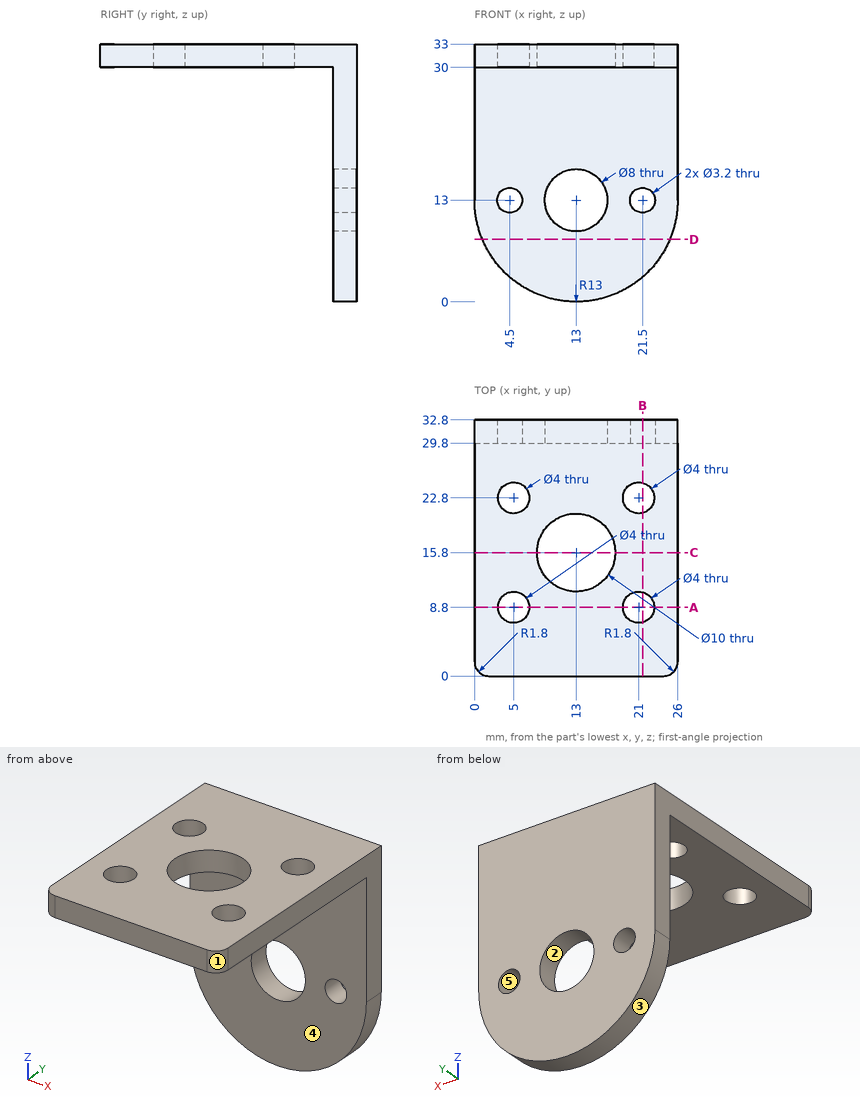
Check sheet for the drawn part. Datum: minimum x, y, z corner. Units: mm. A direction names the side the tool comes from. Coordinates: 2 decimals unless noted, no trailing zeros. Order: outer loops, then holes, each group sorted by start corner. A loop starts at its lowest first (then second) coordinate and runs counter-clockwise, first axis right, second up. Notation, with made-up numbers: M 75.5,-10.5 L 98.5,-10.5 A34 cw 98.5,23.5 Z; hole C 52,6.5 d8. An arc over 180 degrees is marked long. One line per question, with ' | ' between items. Start each with the question number.
Item 1: Access from +Z, -Z, +X, -X, +Y, -Y to the whole of each face (thin tool, end or side, straight path). Record for the marked faces 4 and 5.
Item 2: Gauge pin test, flat ends, axial feed: P1, Ø3.5, axis at x = 21.5, z = 13, coming from the -Y side; P2, Ø11.5, axis at x = 13, y = 15.8, coming from the -Z side; P3, Ø8, axis at x = 20, y = 28.5, coming from the -Z side. Record the tip position at first contact, or that the pin passes through.
Item 3: Sectioned sample at A-A on y = 8.8. Record the cut outline in (x, z).
Item 4: Mould release check, pull along Z, two halves, no side actions. Record for the marked faces 1, 2 and 3: pulls with the +Z half, pulls with the -Z half, needs draft (parallel to the pull), parting line crosses it, or undercut.
Item 5: Sectioned sample at C-C on y = 15.8. Record the cut outline in (x, z), and give its area (3 significant figures).
Item 6: Sectioned sample at B-B on x = 21.5. Record the cut outline in (y, z).
Item 7: Material ranges on line 1 (Y direction, x = 5, z = 32.3); line 2 (Y direction, x = 13, z = 30.75); line 3 (X direction, y = 8, z = 32), recorded low to high.
Item 8: Sectioned sample at D-D on z = 8. Record the cut outline in (x, y).
Answer below:
1) face 4: -Z, +X, -X, -Y | face 5: +Y, -Y
2) P1: stops at y = 29.8 | P2: stops at z = 30 | P3: stops at z = 0.4
3) outline: M 0,30 L 3,30 L 3,33 L 0,33 Z; M 7,30 L 19,30 L 19,33 L 7,33 Z; M 23,30 L 26,30 L 26,33 L 23,33 Z
4) face 1: needs draft | face 2: undercut | face 3: pulls with the -Z half
5) outline: M 0,30 L 8,30 L 8,33 L 0,33 Z; M 18,30 L 26,30 L 26,33 L 18,33 Z | area: 48.0 mm^2
6) outline: M 0,30 L 6.86,30 L 6.86,33 L 0,33 Z; M 10.74,30 L 20.86,30 L 20.86,33 L 10.74,33 Z; M 24.74,30 L 29.8,30 L 29.8,14.6 L 32.8,14.6 L 32.8,33 L 24.74,33 Z; M 29.8,3.16 L 32.8,3.16 L 32.8,11.4 L 29.8,11.4 Z
7) line 1: y = 0 to 6.8, 10.8 to 20.8, 24.8 to 32.8 | line 2: y = 0 to 10.8, 20.8 to 32.8 | line 3: x = 0 to 3.17, 6.83 to 19.17, 22.83 to 26
8) outline: M 1,29.8 L 25,29.8 L 25,32.8 L 1,32.8 Z
